Verification items for the finished model (mm, model axes). A direction names the side the tool comes from. Round coordinates to 2 decimals unless told otherwise and drop trailing zeros. Write each loop counter-clockwise with the first axis right and the second up, starting at its lowest first coordinate (ties: lowest second). Pieces come first, ordered by that corner, then holes. Notation, with made-up numbers: M -31.75,21.25 L 24.25,21.25 A11 ccw 24.25,28.25 Z; hole C -13.75,82.5 d4. An arc over 180 degrees is marked long. Answer in a Markdown table with one row per item. Add a question column.
1. Material ranges on probe 1 along Y at (x, z) = (0, 1); probe 2 along Z at (x, y) = (-3, 5.5); probe 3 along Y at (x, z) = (30.5, 4.25), recorded low to high.
2. Sectioned sample at B-B on y = 0. Record the cut outline in (x, z).
3. Sectioned sample at D-D on z = 5.5. Record the cut outline in (x, y).
4. Set-up check for faces 1 (the cylindrical face through (-34.77, 0.08, 1.52)), 2 (the flat face through (30, -4, 6)), 3 (the cylindrical face through (-30.156, -2.009, 4.979)): record each of +Z, -Z, +X, -X, +Y, -Y from which the full face is reachable in a straight line by a thin tool's end or side.
5. Sectioned sample at A-A on x = 0. Record the cut outline in (y, z).
6. Go/stop test with flat-tipped pins: pin 1 Ø1.9 at (y, z) = (3, 6.5) entering from +X; pin 2 Ø1.9 at (y, z) = (-4, 5) entering from +X; pin 3 Ø4 at (x, y) = (17, 0.5) entering from +Z. Record where each tip stops, or that it passes through.
7. Sectioned sample at C-C on y = -4.75. Record the cut outline in (x, z).
Autodesk Inventor part; units mm, degrees
ref_plane "YZ Plane" through (0, 0, 0) normal (1, 0, 0) x (0, 1, 0)
ref_plane "XZ Plane" through (0, 0, 0) normal (0, 1, 0) x (-1, 0, 0)
ref_plane "XY Plane" through (0, 0, 0) normal (0, 0, 1) x (1, 0, 0)
sketch "Sketch1" plane through (0, 0, 0) normal (0, 0, 1) x (1, 0, 0)
  line L0 (-36, 5.9) -> (36, 5.9)
  line L1 (36, 5.9) -> (36, -5.9)
  line L2 (36, -5.9) -> (-36, -5.9)
  line L3 (-36, -5.9) -> (-36, 5.9)
  line L4 (-30, 5.9) -> (-30, -5.9)
  line L5 (30, 5.9) -> (30, -5.9)
  point P0 (0, 0)
  point P1 (0, 5.9)
  point P2 (-36, 0)
  dimension "d0" = 11.8
  dimension "d1" = 72
  dimension "d2" = 6
  dimension "d3" = 6
extrude "Extrusion1" add sketch "Sketch1" along normal blind 4.2
extrude "Extrusion2" add sketch "Sketch1" along normal blind 8 contours L0 L4 L2 L3 | L0 L1 L2 L5
sketch "Sketch2" plane through (0, 0, 8) normal (0, 0, 1) x (1, 0, 0)
  circle A0 centre (-33.022, 0) radius 3.5
  circle A1 centre (-33.022, 0) radius 1.75
  circle A2 centre (0, 0) radius 1.6
  line L0 (0, 3.25) -> (0, 0) construction
  circle A3 centre (33.022, 0) radius 3.5
  circle A4 centre (33.022, 0) radius 1.75
  dimension "d9" = 7
  dimension "d10" = 33.022
  dimension "d11" = 3.5
  dimension "d12" = 3.2
extrude "Extrusion3" cut sketch "Sketch2" against normal up to surface (8 mm away) contours A1 | A2 | A4
chamfer "Chamfer1" distance 4 angle 45 2 edges at (-36, 0, 8) (36, 0, 8)
extrude "Extrusion4" cut sketch "Sketch2" against normal blind 5 contours A0 | A3
properties part number "GA_FixaBase"
Geometry check:
| question | item | result |
|---|---|---|
| 1 | probe 1 | y = -5.9 to -1.6, 1.6 to 5.9 |
| 1 | probe 2 | z = 0 to 4.2 |
| 1 | probe 3 | y = -5.9 to -2.43, 2.43 to 5.9 |
| 2 | outline | M -36,0 L -34.77,0 L -34.77,3 L -36,3 Z; M -31.27,0 L -1.6,0 L -1.6,4.2 L -29.52,4.2 L -29.52,3 L -31.27,3 Z; M 1.6,0 L 31.27,0 L 31.27,3 L 29.52,3 L 29.52,4.2 L 1.6,4.2 Z; M 34.77,0 L 36,0 L 36,3 L 34.77,3 Z |
| 3 | outline | M -34.5,-5.9 L -30,-5.9 L -30,-1.77 A3.5 cw -34.5,-3.17 Z; M -34.5,3.17 A3.5 cw -30,1.77 L -30,5.9 L -34.5,5.9 Z; M 30,-5.9 L 34.5,-5.9 L 34.5,-3.17 A3.5 cw 30,-1.77 Z; M 30,1.77 A3.5 cw 34.5,3.17 L 34.5,5.9 L 30,5.9 Z |
| 4 | face 1 | +Z, -Z |
| 4 | face 2 | +Z, +Y, -Y |
| 4 | face 3 | +Z |
| 5 | outline | M -5.9,0 L -1.6,0 L -1.6,4.2 L -5.9,4.2 Z; M 1.6,0 L 5.9,0 L 5.9,4.2 L 1.6,4.2 Z |
| 6 | pin 1 | stops at x = 34.43 |
| 6 | pin 2 | stops at x = 35.95 |
| 6 | pin 3 | stops at z = 4.2 |
| 7 | outline | M -36,0 L 36,0 L 36,4 L 32,8 L 30,8 L 30,4.2 L -30,4.2 L -30,8 L -32,8 L -36,4 Z |
